from build123d import *

# Parameters (mm, degrees)
BOSS_EXTRUDE1_DEPTH = 3.175
FILLET1_R           = 6.096


with BuildPart() as part:
    # Sketch1 → Boss-Extrude1 (new body)
    with BuildSketch(Plane.XY):
        with BuildLine():
            Line((-66.675, 42.8625), (-35.179, 42.8625))
            ThreePointArc((-35.179, 42.8625), (-23.953679849, 47.512179849), (-19.304, 58.7375))
            Line((-19.304, 58.7375), (-19.304, 131.7625))
            ThreePointArc((-19.304, 131.7625), (-27.305, 139.7635), (-35.306, 131.7625))
            Line((-35.306, 131.7625), (-35.306, 125.4125))
            Line((-35.306, 125.4125), (-48.006, 125.4125))
            Line((-48.006, 125.4125), (-48.006, 131.7625))
            ThreePointArc((-48.006, 131.7625), (-27.305, 152.4635), (-6.604, 131.7625))
            Line((-6.604, 131.7625), (-6.604, 58.7375))
            ThreePointArc((-6.604, 58.7375), (-1.954320151, 47.512179849), (9.271, 42.8625))
            Line((9.271, 42.8625), (19.431, 42.8625))
            ThreePointArc((19.431, 42.8625), (30.656320151, 47.512179849), (35.306, 58.7375))
            Line((35.306, 58.7375), (35.306, 131.7625))
            ThreePointArc((35.306, 131.7625), (27.305, 139.7635), (19.304, 131.7625))
            Line((19.304, 131.7625), (19.304, 125.4125))
            Line((19.304, 125.4125), (6.604, 125.4125))
            Line((6.604, 125.4125), (6.604, 131.7625))
            ThreePointArc((6.604, 131.7625), (27.305, 152.4635), (48.006, 131.7625))
            Line((48.006, 131.7625), (48.006, 58.7375))
            ThreePointArc((48.006, 58.7375), (52.655679849, 47.512179849), (63.881, 42.8625))
            Line((63.881, 42.8625), (66.675, 42.8625))
            ThreePointArc((66.675, 42.8625), (73.410192091, 40.072692091), (76.2, 33.3375))
            Line((76.2, 33.3375), (76.2, -33.3375))
            ThreePointArc((76.2, -33.3375), (73.410192091, -40.072692091), (66.675, -42.8625))
            Line((66.675, -42.8625), (-66.675, -42.8625))
            ThreePointArc((-66.675, -42.8625), (-73.410192091, -40.072692091), (-76.2, -33.3375))
            Line((-76.2, -33.3375), (-76.2, 33.3375))
            ThreePointArc((-76.2, 33.3375), (-73.410192091, 40.072692091), (-66.675, 42.8625))
        make_face()
        with BuildLine():
            Line((-57.785, 26.9875), (57.785, 26.9875))
            ThreePointArc((57.785, 26.9875), (59.581051224, 26.243551224), (60.325, 24.4475))
            Line((60.325, 24.4475), (60.325, -24.4475))
            ThreePointArc((60.325, -24.4475), (59.581051224, -26.243551224), (57.785, -26.9875))
            Line((57.785, -26.9875), (-57.785, -26.9875))
            ThreePointArc((-57.785, -26.9875), (-59.581051224, -26.243551224), (-60.325, -24.4475))
            Line((-60.325, -24.4475), (-60.325, 24.4475))
            ThreePointArc((-60.325, 24.4475), (-59.581051224, 26.243551224), (-57.785, 26.9875))
        make_face(mode=Mode.SUBTRACT)
    extrude(amount=BOSS_EXTRUDE1_DEPTH)

    # Fillet1
    fillet1_edges = [part.edges().sort_by_distance(p)[0] for p in [
        (-35.306, 125.4125, 1.5875),
        (-48.006, 125.4125, 1.5875),
        (19.304, 125.4125, 1.5875),
        (6.604, 125.4125, 1.5875),
    ]]
    fillet(fillet1_edges, radius=FILLET1_R)


solid = part.part
Here's how the part is built. I have some questions about the finished solid (model axes, mm). A direction names the side the tool comes from. Coordinates: 2 decimals unless noted, no trailing zeros. Loops run counter-clockwise (first coordinate to the right, second up) from the corner with the lowest first, then second, coordinate; pieces in that order, holes last.
1. Imagine slicing it at A-A, the plane y = -5.5. Please give me the cut outline in (x, z) (3 decimals).
2. For P1, Ø1, axis at x = 12.5, z = 2, coming from the +Y side; P2, Ø1.6, axis at x = -46, z = 1, coming from the +Y side; P3, Ø1, axis at y = 109, z = 1.5, coming from the +X side, each with a flat end and sliding along its axis, tell me the tip position at first contact or that it passes through.
3. I need wall thicknesses on L1, parallel to X at y = 10, z = 1.7 (3 decimals); L2, parallel to X at y = 99, z = 1.45; L3, parallel to Y at x = 32.5, z = 2. Which ranges of each line are inside material? Lowest first, please.
4. Imagine slicing it at B-B, the plane x = 16. Please give me the cut outline in (y, z) (1 decimal), and give its area (3 significant figures).
5. For faces 1 (the cylindrical face through (8.34, 127.25, 1.61)), 2 (the flat face through (1, 34, 3.175)), 3 (the cylindrical face through (-46.17, 127.15, 1.61)), which set-ups out of +Z, -Z, +X, -X, +Y, -Y let a thin tool reach every point of the face, with its end or its side?
6. Imagine slicing it at D-D, the plane y = 71. Please give me the cut outline in (x, z) (3 decimals).
7. Imagine slicing it at C-C, the plane y = 128.5. Please give me the cut outline in (x, z) (3 decimals), and give its area (3 significant figures).
8. If we mould it in two halves opening along X, with no side actions, what happens to faces 4 (the cylindrical face through (73.48, -40, 1.57)), 5 (the cylindrical face through (17.47, 127.15, 1.61)), 6 (the cylindrical face through (-73.48, 40, 1.57))? For each: pulls with the +X half, pulls with the -X half, needs draft (parallel to the pull), parting line crosses it, or undercut.
Taken from the geometry:
1. outline: (-76.2, 0) - (-60.325, 0) - (-60.325, 3.175) - (-76.2, 3.175) - close; (60.325, 0) - (76.2, 0) - (76.2, 3.175) - (60.325, 3.175) - close
2. P1: stops at y = 146.73
2. P2: stops at y = 142.17
2. P3: stops at x = 48.01
3. L1: x = -76.2 to -60.325, 60.325 to 76.2
3. L2: x = -19.3 to -6.6, 35.31 to 48.01
3. L3: y = -42.86 to -26.99, 26.99 to 49.73, 137.85 to 151.8
4. outline: (-42.9, 0) - (-27, 0) - (-27, 3.2) - (-42.9, 3.2) - close; (27, 0) - (42.9, 0) - (42.9, 3.2) - (27, 3.2) - close; (126.1, 0) - (149.1, 0) - (149.1, 3.2) - (126.1, 3.2) - close
4. area: 174 mm2
5. face 1: +Z, -Z
5. face 2: +Z, +X, -X, +Y, -Y
5. face 3: +Z, -Z, -X
6. outline: (-19.304, 0) - (-6.604, 0) - (-6.604, 3.175) - (-19.304, 3.175) - close; (35.306, 0) - (48.006, 0) - (48.006, 3.175) - (35.306, 3.175) - close
7. outline: (-47.212, 0) - (-36.1, 0) - (-36.1, 3.175) - (-47.212, 3.175) - close; (-19.304, 0) - (-6.604, 0) - (-6.604, 3.175) - (-19.304, 3.175) - close; (7.398, 0) - (18.51, 0) - (18.51, 3.175) - (7.398, 3.175) - close; (35.306, 0) - (48.006, 0) - (48.006, 3.175) - (35.306, 3.175) - close
7. area: 151 mm2
8. face 4: pulls with the +X half
8. face 5: undercut
8. face 6: pulls with the -X half
